Solid Edge part; units mm, degrees
sketch "Sketch1" plane through (10.8674, 0, 10.8674) normal (0, -1, 0) x (1, 0, 0)
  line L0 (-19.8674, -10.8674) -> (-19.8674, -4.1174)
  line L1 (-19.8674, -4.1174) -> (-11.8674, -4.1174)
  line L2 (-11.8674, -4.1174) -> (-11.8674, -6.8674)
  line L3 (-11.8674, -6.8674) -> (-1.8674, -6.8674)
  line L4 (-1.8674, -6.8674) -> (-1.8674, -10.8674)
revolve "RevolvedProtrusion1" add sketch "Sketch1" angle 360 about axis through (16.5, 0, 0) along (-1, 0, 0)
sketch "Sketch2" plane through (-9, 0, 0) normal (-1, 0, 0) x (0, 0, -1)
  line L0 (4.6188, 0) -> (2.3094, 4)
  line L1 (2.3094, 4) -> (-2.3094, 4)
  line L2 (-2.3094, 4) -> (-4.6188, 0)
  line L3 (-4.6188, 0) -> (-2.3094, -4)
  line L4 (-2.3094, -4) -> (2.3094, -4)
  line L5 (2.3094, -4) -> (4.6188, 0)
extrude "Cutout1" cut sketch "Sketch2" against normal blind 4
cosmetic_thread "Gänga" thread depth 5
properties material "Steel"
Geometry check sheet. Reference: the model listing, model coordinates, mm. A direction names the side the tool comes from. Round coordinates to 2 decimals unless told otherwise and drop trailing zeros. Loops run counter-clockwise (first coordinate to the right, second up) from the corner with the lowest first, then second, coordinate; pieces in that order, holes last. Notation, with made-up numbers: M 86,72.5 L 94,72.5 A23 cw 94,99.5 Z; hole C 67.25,84.5 d2. An arc over 180 degrees is marked long. Return JSON: item names as keys, results as strings. Group by question number.
(1) Section check C-C, the plane x = 0. Enter the section's corners in (y, z).
(2) Go/stop test with flat-tipped pins: pin 1 (5 mm diameter, centred on y = -4.5, z = 5.5, fed in from +X); pin 2 (4 mm diameter, centred on x = 0, z = 2, fed in from +Y); pin 3 (6 mm diameter, centred on x = 6, y = -1.5, fed in from -Z). Record where each tip stops, or that it passes through.
(3) Section check B-B, the plane y = 3.25. Enter the section's corners in (x, z).
(4) Set-up check for faces 4 (the face through (-1, -3, 3)), 5 (the face through (-9, -4.4, -0.1)), 6 (the face through (-7.028, 2.028, -3.448)): record each of +Z, -Z, +X, -X, +Y, -Y from which the full face is reachable in a straight line by a thin tool's end or side.
(5) Scan lines: line 1 along X through (y, z) = (1.25, 6); line 2 along Y through (x, z) = (1.5, 0); line 3 along X through (y, z) = (0, 4.5). Record each from-to range of solid material in increasing order. Write a range as [from, to].
(6) Section check A-A, the plane z = 0. Enter the section's corners in (x, y), and give its area (3 significant figures).
(7) Mould release check, pull along Z, two halves, no side actions. Record for faces 1 (the face through (-4.94, 6.59, -1.46)), 2 (the face through (9, 0, 0)), 3 (the face through (-7.028, -2.028, 3.448)): pulls with the +Z half, pulls with the -Z half, needs draft (parallel to the pull), parting line crosses it, or undercut.
Data:
{
 "1": {"outline": "C 0,0 d8"},
 "2": {"pin 1": "x = -1", "pin 2": "y = 6.74", "pin 3": "z = -4"},
 "3": {"outline": "M -9,-5.92 L -1,-5.92 L -1,-2.33 L 9,-2.33 L 9,2.33 L -1,2.33 L -1,5.92 L -9,5.92 L -9,2.74 L -5,2.74 L -5,-2.74 L -9,-2.74 Z"},
 "4": {"face 4": "+X", "face 5": "+Z, -Z, -X, +Y, -Y", "face 6": "-X"},
 "5": {"line 1": "[-9, -1]", "line 2": "[-4, 4]", "line 3": "[-5, -1]"},
 "6": {"outline": "M -9,-6.75 L -1,-6.75 L -1,-4 L 9,-4 L 9,4 L -1,4 L -1,6.75 L -9,6.75 L -9,4 L -5,4 L -5,-4 L -9,-4 Z", "area": "156 mm²"},
 "7": {"face 1": "parting line crosses it", "face 2": "needs draft", "face 3": "undercut"}
}
